Design review of the part built by this model. Coordinates are the model's own, in mm. A direction names the side the tool comes from. Give positions to 0.01 mm unless a question says otherwise; leave off trailing zeros. Loops run counter-clockwise (first coordinate to the right, second up) from the corner with the lowest first, then second, coordinate; pieces in that order, holes last. Notation, with made-up numbers: (13, 2.25) -> (29, 2.25) arc R19 ccw to (29, 18.25) -> close; hole circle Ø1 at (-21, 47.25). An arc over 180 degrees is marked (long way). Answer in a Markdown table with one row per item. Add a question column.
(1) For line 1 (X direction, y = -0.25, z = -37); line 2 (Z direction, x = 1, y = -0.6); line 3 (X direction, y = -2.3, z = -35.5), list the stretches that pass through material, from the lowest coordinate up.
(2) For pin 1 (3 mm diameter, centred on x = -40.64, z = -36.322, fed in from +Y); pin 2 (4 mm diameter, centred on x = 40.64, z = -36.322, fed in from -Y) (3 decimals); pin 3 (1.6 mm diameter, centred on x = 54.5, y = -2, fed in from +Z), all flat-tipped, find the tip position at first contact; note any pin that passes through.
(3) Consider section A-A on x = 0. Write out the cut boundary in (y, z) (3 decimals).
(4) Consider section C-C on y = -2.3. Write out the cut boundary in (x, z), then the cut area to 3 significant figures.
(5) Consider section B-B on x = 40.64. Write out the cut boundary in (y, z) (3 decimals).
(6) Consider section D-D on x = -30.5. Write out the cut boundary in (y, z) (3 decimals), then the cut area to 3 significant figures.
(7) Draft analysis for pull direction X (two halves, no side actions). For faces 1 (the flat face through (40, -2, 23.622)), 2 (the flat face through (74.676, -2, -9)), 3 (the cylindrical face through (-40.57, -1.57, -37.97)), 4 (the cylindrical face through (0.089, -1.565, -38.352)), state which applies: +X half, -X half, draft (parallel to the pull), parting line (faces both ways), or undercut.
(8) For faces 5 (the cylindrical face through (0.5, -1.57, 41.45)), 6 (the flat face through (3.81, -2, 36)), 7 (the flat face through (-3.81, -2, 36)), list the 3-axis set-ups (+Z, -Z, +X, -X, +Y, -Y) from which the entire face can be reached by the end or side of a thin tool; tool diameter is ignored.
from build123d import *

# Parameters (mm, degrees)
BOSS_EXTRUDE1_DEPTH = 3.175
SKETCH2_R           = 1.651
SKETCH2_R_2         = 2.032
CUT_EXTRUDE1_DEPTH  = 89.969731937


with BuildPart() as part:
    # Sketch1 → Boss-Extrude1 (new body)
    with BuildSketch(Plane(origin=(0, 0, 0), x_dir=(1, 0, 0), z_dir=(0, 1, 0))):
        Polygon((-74.676, 41.402), (74.676, 41.402), (74.676, -23.622), (3.81, -23.622), (3.81, -48.26), (-3.81, -48.26), (-3.81, -23.622), (-74.676, -23.622), align=None)
    extrude(amount=-BOSS_EXTRUDE1_DEPTH)

    # Sketch2 → Cut-Extrude1 (cut, through all)
    with BuildSketch(Plane(origin=(0, 0, 0), x_dir=(1, 0, 0), z_dir=(0, 1, 0))):
        with Locations(Location((-40.64, 36.322, 0), (0, 0, 270))):
            Circle(SKETCH2_R)
        with Locations(Location((0, 36.322, 0), (0, 0, 270))):
            Circle(SKETCH2_R_2)
        with Locations(Location((40.64, 36.322, 0), (0, 0, 270))):
            Circle(SKETCH2_R)
        with Locations(Location((0, -39.878, 0), (0, 0, 270))):
            Circle(SKETCH2_R)
    extrude(amount=-CUT_EXTRUDE1_DEPTH, mode=Mode.SUBTRACT)


solid = part.part
Values follow:
| question | item | result |
|---|---|---|
| 1 | line 1 | -74.68 to -42.15, -39.13 to -1.92, 1.92 to 39.13, 42.15 to 74.68 |
| 1 | line 2 | -41.4 to -38.09, -34.55 to 38.56, 41.19 to 48.26 |
| 1 | line 3 | -74.68 to -42.07, -39.21 to -1.86, 1.86 to 39.21, 42.07 to 74.68 |
| 2 | pin 1 | through |
| 2 | pin 2 | y = -3.175 |
| 2 | pin 3 | z = 23.62 |
| 3 | outline | (-3.175, -41.402) -> (0, -41.402) -> (0, -38.354) -> (-3.175, -38.354) -> close; (-3.175, -34.29) -> (0, -34.29) -> (0, 38.227) -> (-3.175, 38.227) -> close; (-3.175, 41.529) -> (0, 41.529) -> (0, 48.26) -> (-3.175, 48.26) -> close |
| 4 | outline | (-74.68, -41.4) -> (74.68, -41.4) -> (74.68, 23.62) -> (3.81, 23.62) -> (3.81, 48.26) -> (-3.81, 48.26) -> (-3.81, 23.62) -> (-74.68, 23.62) -> close; hole circle Ø3.3 at (-40.64, -36.32); hole circle Ø4.06 at (0, -36.32); hole circle Ø3.3 at (0, 39.88); hole circle Ø3.3 at (40.64, -36.32) |
| 4 | area | 9,860 mm2 |
| 5 | outline | (-3.175, -41.402) -> (0, -41.402) -> (0, -37.973) -> (-3.175, -37.973) -> close; (-3.175, -34.671) -> (0, -34.671) -> (0, 23.622) -> (-3.175, 23.622) -> close |
| 6 | outline | (-3.175, -41.402) -> (0, -41.402) -> (0, 23.622) -> (-3.175, 23.622) -> close |
| 6 | area | 206 mm2 |
| 7 | face 1 | draft |
| 7 | face 2 | +X half |
| 7 | face 3 | undercut |
| 7 | face 4 | undercut |
| 8 | face 5 | +Y, -Y |
| 8 | face 6 | +Z, +X, +Y, -Y |
| 8 | face 7 | +Z, -X, +Y, -Y |
